Geometry check sheet. Reference: the model listing, model coordinates, mm. A direction names the side the tool comes from. Give positions to 0.01 mm unless a question says otherwise; leave off trailing zeros. Loops run counter-clockwise (first coordinate to the right, second up) from the corner with the lowest first, then second, coordinate; pieces in that order, holes last. Notation, with made-up numbers: (2.5, -29) - (44.5, -29) arc R26 cw to (44.5, 1) - close; hole circle Ø4 at (-12.5, 2). An arc over 180 degrees is marked (long way). Use a Markdown table: item, result. Add a question column.
1. Draft check along Z on faces 1 (the flat face through (167, 30, -42.68)), 2 (the flat face through (165, 24.181, 2)), 3 (the flat face through (58, 26, 69.588)), 4 (the flat face through (-54.229, 26, 13)). Enter one of: pulls with the +Z half, pulls with the -Z half, needs draft (parallel to the pull), parting line crosses it, or undercut.
2. Depth check by flat-ended pin: P1, Ø5, axis at y = 41, z = 51, coming from the +X side; P2, Ø21, axis at y = 32.5, z = -12.5, coming from the +X side; P3, Ø6.5, axis at x = 163.5, z = -3, coming from the +Y side. Enter the tip coordinate at first touch or a pass-through.
3. Set-up check for faces 5 (the flat face through (59, 0, 12)), 6 (the flat face through (167, 9.195, 56)): record each of +Z, -Z, +X, -X, +Y, -Y from which the full face is reachable in a straight line by a thin tool's end or side.
4. Material ranges on L1, parallel to X at y = 46.5, z = 15, recorded low to high.
5. Cross-section at B-B on y = 45.5. Enter the section's corners in (x, z).
6. Cross-section at C-C on z = 19.5. Enter the section's corners in (x, y).
7. Cross-section at A-A on z = 61. Enter the section's corners in (x, y), and give its area (3 significant figures).
from build123d import *

# Parameters (mm, degrees)
SKETCH1_W           = 228.6
SKETCH1_H           = 114.3
BOSS_EXTRUDE1_DEPTH = 50.8
SKETCH2_W           = 15.24
SKETCH2_H           = 110.236
CUT_EXTRUDE1_DEPTH  = 41.6052
SKETCH3_W           = 15.24
SKETCH3_H           = 86.2584
BOSS_EXTRUDE2_DEPTH = 14.986
FILLET1_R           = 2.54
FILLET2_R           = 1.27
FILLET3_R           = 2.54


with BuildPart() as part:
    # Sketch1 → Boss-Extrude1 (new body)
    with BuildSketch(Plane(origin=(0, 0, 0), x_dir=(1, 0, 0), z_dir=(0, 1, 0))):
        with Locations((60.070744159, -12.437798992)):
            Rectangle(SKETCH1_W, SKETCH1_H)
    extrude(amount=BOSS_EXTRUDE1_DEPTH)

    # Sketch2 → Cut-Extrude1 (cut)
    with BuildSketch(Plane(origin=(0, 50.8, 0), x_dir=(1, 0, 0), z_dir=(0, 1, 0))):
        with Locations((166.750744159, -12.437798992)):
            Rectangle(SKETCH2_W, SKETCH2_H)
    extrude(amount=-CUT_EXTRUDE1_DEPTH, mode=Mode.SUBTRACT)

    # Sketch3 → Boss-Extrude2 (add)
    with BuildSketch(Plane(origin=(0, 9.1948, 0), x_dir=(1, 0, 0), z_dir=(0, 1, 0))):
        with Locations((166.750744159, -2.328598992)):
            Rectangle(SKETCH3_W, SKETCH3_H)
    extrude(amount=BOSS_EXTRUDE2_DEPTH)

    # Fillet1
    fillet1_edges = [part.edges().sort_by_distance(p)[0] for p in [
        (174.370744159, 24.1808, 2.328598992),
    ]]
    fillet(fillet1_edges, radius=FILLET1_R)

    # Fillet2
    fillet2_edges = [part.edges().sort_by_distance(p)[0] for p in [
        (174.370744159, 50.8, 68.571798992),
        (174.370744159, 50.8, -43.696201008),
    ]]
    fillet(fillet2_edges, radius=FILLET2_R)

    # Fillet3
    fillet3_edges = [part.edges().sort_by_distance(p)[0] for p in [
        (60.070744159, 0, -44.712201008),
        (174.370744159, 0, 12.437798992),
        (60.070744159, 0, 69.587798992),
        (-54.229255841, 0, 12.437798992),
    ]]
    fillet(fillet3_edges, radius=FILLET3_R)


solid = part.part
Values found:
| question | item | result |
|---|---|---|
| 1 | face 1 | undercut |
| 1 | face 2 | undercut |
| 1 | face 3 | pulls with the +Z half |
| 1 | face 4 | needs draft |
| 2 | P1 | stops at x = 159.13 |
| 2 | P2 | stops at x = 174.35 |
| 2 | P3 | stops at y = 24.18 |
| 3 | face 5 | +Z, -Z, +X, -X, -Y |
| 3 | face 6 | +X, +Y |
| 4 | L1 | x = -54.23 to 159.13 |
| 5 | outline | (-54.23, -44.71) - (174.37, -44.71) - (174.37, -42.68) - (159.13, -42.68) - (159.13, 67.56) - (174.37, 67.56) - (174.37, 69.59) - (-54.23, 69.59) - close |
| 6 | outline | (-54.23, 2.54) arc R2.54 ccw to (-51.69, 0) - (171.83, 0) arc R2.54 ccw to (174.37, 2.54) - (174.37, 21.64) arc R2.54 ccw to (171.83, 24.18) - (159.13, 24.18) - (159.13, 50.8) - (-54.23, 50.8) - close |
| 7 | outline | (-54.23, 2.54) arc R2.54 ccw to (-51.69, 0) - (171.83, 0) arc R2.54 ccw to (174.37, 2.54) - (174.37, 9.19) - (159.13, 9.19) - (159.13, 50.8) - (-54.23, 50.8) - close |
| 7 | area | 11,000 mm2 |
